```python
from build123d import *

# Parameters (mm, degrees)
SKETCH2_W          = 56.9
SKETCH2_H          = 218.001042519
SKETCH3_R          = 54.081739793
CUT_EXTRUDE1_DEPTH = 210
FILLET1_R          = 10


with BuildPart() as part:
    # Sketch2 → Revolve2 (revolve)
    with BuildSketch(Plane.XY, mode=Mode.PRIVATE) as revolve2_sk:
        with Locations((321.328943302, 175.938289097)):
            Rectangle(SKETCH2_W, SKETCH2_H)
    revolve(revolve2_sk.sketch.rotate(Axis((349.778943302, 284.938810356, 0), (0, -1, 0)), 270), axis=Axis((349.778943302, 284.938810356, 0), (0, -1, 0)))

    # Sketch3 → Cut-Extrude1 (cut)
    with BuildSketch(Plane(origin=(0, 284.938810356, 0), x_dir=(1, 0, 0), z_dir=(0, 1, 0))):
        with Locations(Location((349.778943302, 0, 0), (0, 0, 270))):
            Circle(SKETCH3_R)
    extrude(amount=-CUT_EXTRUDE1_DEPTH, mode=Mode.SUBTRACT)

    # Fillet1
    fillet1_edges = [part.edges().sort_by_distance(p)[0] for p in [
        (349.778943302, 74.938810356, -54.081739793),
    ]]
    fillet(fillet1_edges, radius=FILLET1_R)


solid = part.part
```
CAD build for the part. Positions are in the model's coordinates, mm. A direction names the side the tool comes from. Give positions to 0.01 mm unless a question says otherwise; leave off trailing zeros. Order: outer loops, then holes, each group sorted by start corner. A loop starts at its lowest first (then second) coordinate and runs counter-clockwise, first axis right, second up. Notation, with made-up numbers: M 22.5,77.25 L 31.5,77.25 A33 ccw 31.5,108.25 Z; hole C 47,-21.75 d1. An arc over 180 degrees is marked long. Put each result on its own line as item: value. Start each with the question number.
(1) Which spindle directions (+Z, -Z, +X, -X, +Y, -Y) get a long thin tool onto all of the face, cutting with end or side? Do faces 4 (the cylindrical face through (403.4, 186.34, -7.04)), 5 (the flat face through (371, 284.939, 50)). Say none if no direction does.
(2) Flat gauge pins, fed straight in: pin 1 Ø2 at (x, z) = (392.5, -41) entering from +Y; pin 2 Ø3 at (x, y) = (383.5, 153) entering from -Z; pin 3 Ø4 at (x, y) = (318, 169.5) entering from -Z; pin 4 Ø1.5 at (x, z) = (377, -37.5) entering from +Y. Where does each tip first touch, or does it go through?
(3) Saw through at A-A, the plane z = 0. Write the cut outline in (x, y), then the cut area to 3 significant figures.
(4) Saw through at B-B, the plane y = 89. Write the cut outline in (x, z).
(5) Drill centre lines: line 1 along Z through (x, y) = (349, 217.5); line 2 along X through (y, z) = (212, -1.5); line 3 along X through (y, z) = (210, 0). Where is each one in solid material? Low to high.
(6) Mould opens along Z. For faces 1 (the flat face through (349, 66.938, -1)), 2 (the flat face through (350, 74.939, -1)), 3 (the cylindrical face through (293.363, 177.464, -7.407)) say: +Z half, -Z half, draft (parallel to the pull), parting line (faces both ways), or undercut.
Check result:
1. face 4: +Y
1. face 5: +Z, -Z, +X, -X, +Y
2. pin 1: passes through
2. pin 2: stops at z = -46.9
2. pin 3: stops at z = -48.49
2. pin 4: stops at y = 75.4
3. outline: M 292.88,66.94 L 406.68,66.94 L 406.68,284.94 L 403.86,284.94 L 403.86,84.94 A10 cw 393.86,74.94 L 305.7,74.94 A10 cw 295.7,84.94 L 295.7,284.94 L 292.88,284.94 Z
3. area: 2,140 mm2
4. outline: C 349.78,0 d113.8; hole C 349.78,0 d108.16
5. line 1: z = -56.89 to -54.08, 54.08 to 56.89
5. line 2: x = 292.9 to 295.72, 403.84 to 406.66
5. line 3: x = 292.88 to 295.7, 403.86 to 406.68
6. face 1: draft
6. face 2: undercut
6. face 3: parting line
